For this review, use the dimensioned drawing (mm, ordinates from the lowest corner) and the shaded views. A direction names the side the tool comes from. Coordinates: 2 decimals unless noted, no trailing zeros. Write each loop counter-clockwise with the first axis right and the second up, starting at its lowest first coordinate (ties: lowest second). Pieces come first, ordered by that corner, then holes. Notation, with made-up numbers: (0, 63.25) - (56, 63.25) arc R12 ccw to (56, 74.25) - close; hole circle Ø6 at (-31, -21.75). An arc over 180 degrees is marked (long way). One line per item, written item: value.
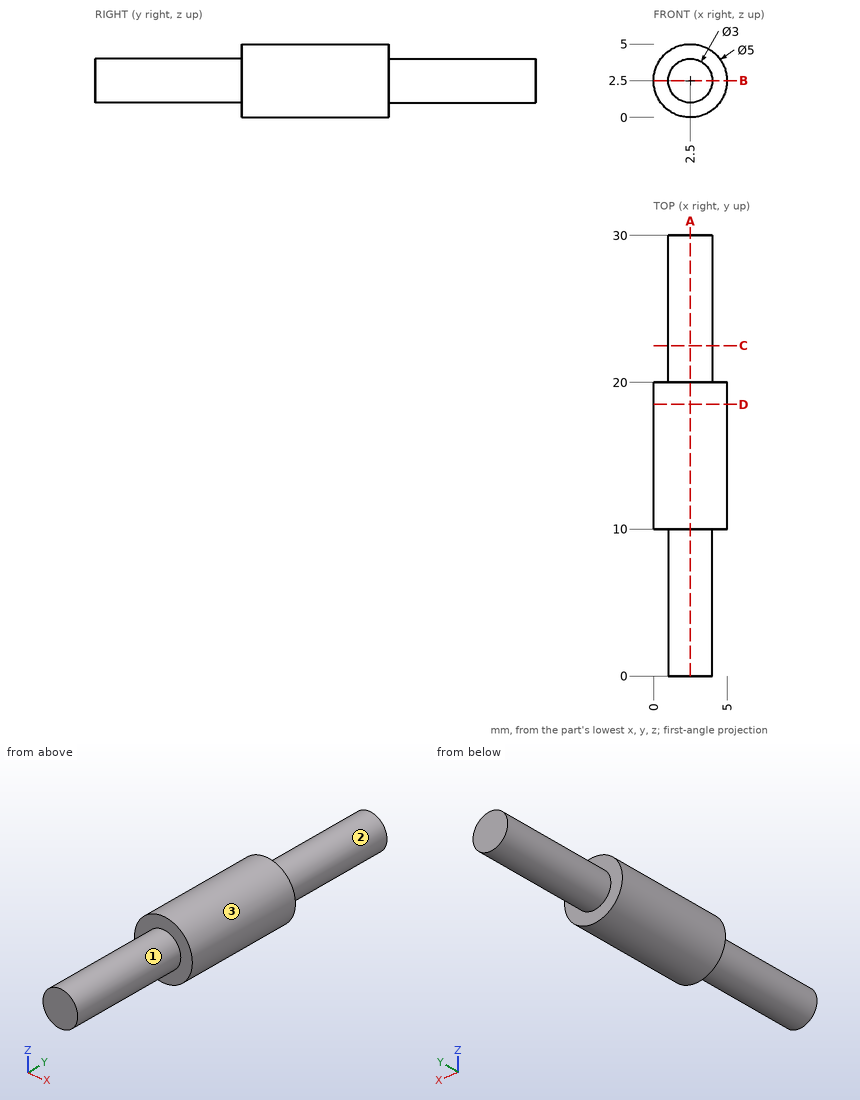
1. Wall thickness on line 1 along Y through (x, z) = (0.45, 2.05); line 2 along X through (y, z) = (6.5, 1.3); line 3 along X through (y, z) = (23, 1.4): over which ranges is each line inside the solid? List them lowest first.
Answer block:
line 1: y = 10 to 20
line 2: x = 1.6 to 3.4
line 3: x = 1.48 to 3.52
2. Consider section D-D, the plane y = 18.5. Write out the cut boundary in (x, z), then the cut area to 3 significant figures.
Answer block:
outline: circle Ø5 at (2.5, 2.5)
area: 19.6 mm^2
3. For the marked faces 1, 2 and 3, list the 3-axis set-ups (+Z, -Z, +X, -X, +Y, -Y) from which the entire face can be reached by the end or side of a thin tool; tool diameter is ignored.
Answer block:
face 1: -Y
face 2: +Y
face 3: +Y, -Y
4. Consider section B-B, the plane z = 2.5. Write out the cut boundary in (x, y).
Answer block:
outline: (0, 10) - (1, 10) - (1, 0) - (4, 0) - (4, 10) - (5, 10) - (5, 20) - (4, 20) - (4, 30) - (1, 30) - (1, 20) - (0, 20) - close
5. Consider section C-C, the plane y = 22.5. Write out the cut boundary in (x, z), then the cut area to 3 significant figures.
Answer block:
outline: circle Ø3 at (2.5, 2.5)
area: 7.07 mm^2
6. Insertion check: pin 1 Ø1 at (y, z) = (23.5, 4) entering from +X; pin 2 Ø1 at (x, y) = (1.5, 27) entering from -Z. Each pin has a flat end and moves straight along its axis. Give the tip position at first contact, or say it passes through.
Answer block:
pin 1: stops at x = 3.62
pin 2: stops at z = 1.09
7. Consider section A-A, the plane x = 2.5. Write out the cut boundary in (y, z).
Answer block:
outline: (0, 1) - (10, 1) - (10, 0) - (20, 0) - (20, 1) - (30, 1) - (30, 4) - (20, 4) - (20, 5) - (10, 5) - (10, 4) - (0, 4) - close
